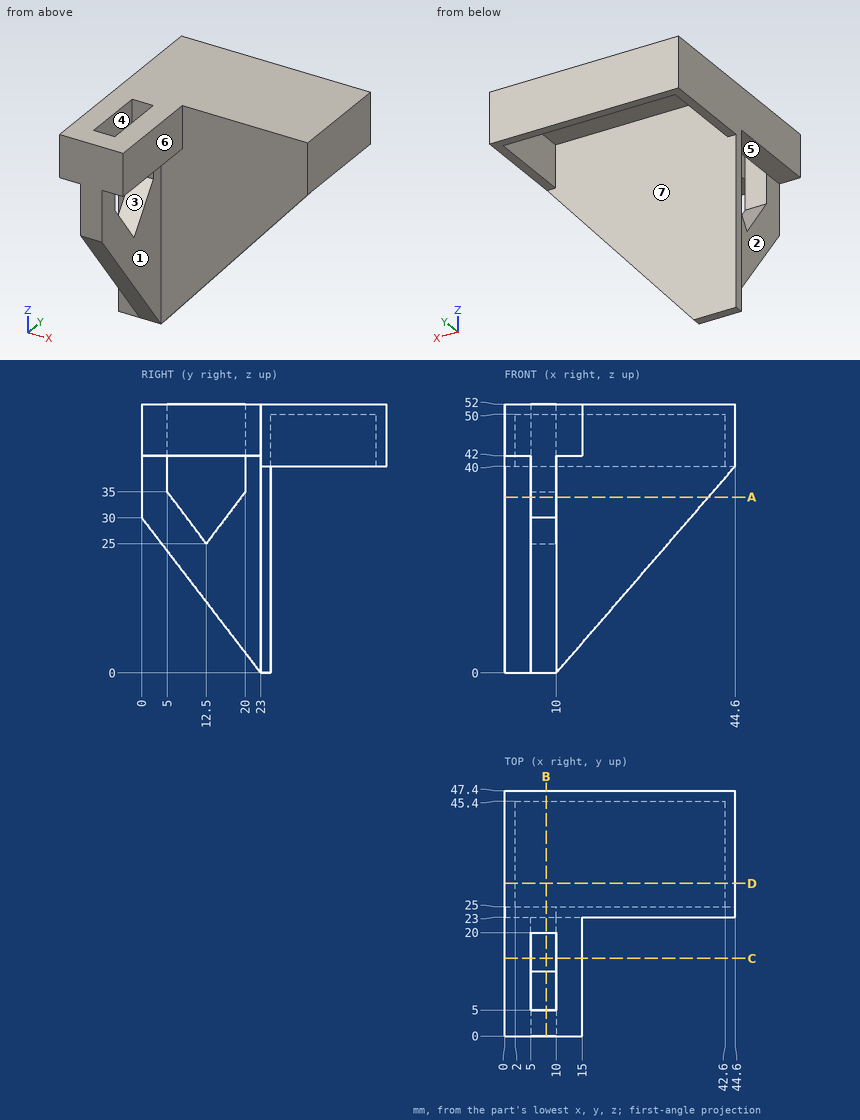
Job drawing, mm, ordinate dimensions from the low corner. One solid piece. A direction names the side the tool comes from. Coordinates: 2 decimals unless noted, no trailing zeros. Write each loop counter-clockwise with the first axis right and the second up, starting at its lowest first coordinate (ties: lowest second). Pieces come first, ordered by that corner, then holes. Notation, with made-up numbers: (52.25, -11) - (101.25, -11) arc R18 cw to (101.25, 20) - close; hole circle Ø4 at (56.5, 44). An arc over 180 degrees is marked (long way). Use a Markdown table: item, result. Add a question column.
Item 1: Band-saw the part on C-C, the plane y = 15. Give the cut face in (x, z), and give its area (3 significant figures).
Item 2: Band-saw the part on D-D, the plane y = 29.5. Give the cut face in (x, z), and give its area (3 significant figures).
Item 3: Mould opens along X. For the marked faces 5, 6 and 7 say: pulls with the +X half, pulls with the -X half, needs draft (parallel to the pull), parting line crosses it, or undercut.
Item 4: Flat gauge pins, fed straight in: pin 1 (3 mm diameter, centred on y = 9, z = 45.5, fed in from +X); pin 2 (2.5 mm diameter, centred on x = 11.5, y = 14.5, fed in from -Z); pin 3 (5 mm diameter, centred on x = 11, z = 36.5, fed in from +Y); pin 4 (5 mm diameter, centred on y = 19.5, z = 44.5, fed in from -X). Where does each tip first touch, or does it go through?
Item 5: Band-saw the part on B-B, the plane x = 8. Give the cut face in (y, z), and give its area (3 significant figures).
Item 6: Band-saw the part on A-A, the plane z = 34. Give the cut face in (x, y).
Item 7: Drill centre lines: L1, parallel to Y at x = 36.5, z = 44.5; L2, parallel to X at y = 28, z = 47.5; L3, parallel to Y at x = 8, z = 36. Where is each one in solid material? Low to high. Write a range as from..to.
Item 8: 3-axis set-ups, long thin cutter, end or side, ignore diameter. For the marked faces 1, 2, 3 and 4: which of +Z, -Z, +X, -X, +Y, -Y reach the whole face in a straight line?
Numbers:
| question | item | result |
|---|---|---|
| 1 | outline | (0, 42) - (5, 42) - (5, 52) - (0, 52) - close; (5, 10.43) - (10, 10.43) - (10, 28.33) - (5, 28.33) - close; (10, 42) - (15, 42) - (15, 52) - (10, 52) - close |
| 1 | area | 189 mm2 |
| 2 | outline | (0, 40) - (2, 40) - (2, 50) - (42.6, 50) - (42.6, 40) - (44.6, 40) - (44.6, 52) - (0, 52) - close |
| 2 | area | 129 mm2 |
| 3 | face 5 | needs draft |
| 3 | face 6 | pulls with the +X half |
| 3 | face 7 | undercut |
| 4 | pin 1 | x = 15 |
| 4 | pin 2 | z = 42 |
| 4 | pin 3 | y = 25 |
| 4 | pin 4 | x = 0 |
| 5 | outline | (0, 30) - (23, 0) - (25, 0) - (25, 50) - (45.4, 50) - (45.4, 40) - (47.4, 40) - (47.4, 52) - (20, 52) - (20, 35) - (12.5, 25) - (5, 35) - (5, 52) - (0, 52) - close |
| 5 | area | 690 mm2 |
| 6 | outline | (0, 23) - (5, 23) - (5, 19.25) - (10, 19.25) - (10, 23) - (39.41, 23) - (39.41, 25) - (0, 25) - close; (5, 0) - (10, 0) - (10, 5.75) - (5, 5.75) - close |
| 7 | L1 | 23..25, 45.4..47.4 |
| 7 | L2 | 0..2, 42.6..44.6 |
| 7 | L3 | 0..5, 20..25 |
| 8 | face 1 | -Z, +X, -Y |
| 8 | face 2 | -Z, -X, -Y |
| 8 | face 3 | +Z, +X, -X |
| 8 | face 4 | +Z |
